Verification items for the finished model (mm, model axes). A direction names the side the tool comes from. Give positions to 0.01 mm unless a question says otherwise; leave off trailing zeros. Loops run counter-clockwise (first coordinate to the right, second up) from the corner with the lowest first, then second, coordinate; pieces in that order, holes last. Notation, with made-up numbers: (-11, 83.25) -> (38, 83.25) arc R37 cw to (38, 120.25) -> close; hole circle Ø11 at (-27.75, 41.5). An arc over 180 degrees is marked (long way). Answer in a Markdown table with one row per item. Add a question column.
Q1. Release check for a two-part mould opening along Y. For faces 1 (the face through (73, 34, 5)), 2 (the face through (-0.86, 56.6, 5.07)), 3 (the face through (86.2, 12.6, 5)) record: pulls with the +Y half, pulls with the -Y half, needs draft (parallel to the pull), parting line crosses it, or undercut.
Q2. Material ranges on probe 1 along X at (y, z) = (13.5, 2); probe 2 along Y at (x, z) = (-11, 6.9); probe 3 along X at (y, z) = (33.5, 5.5), recorded low to high.
Q3. Section check C-C on z = 8. Enter the section's corners in (x, y).
Q4. Section check D-D on z = 1.5. Enter the section's corners in (x, y).
Q5. Gauge pin test, flat ends, axial feed: P1, Ø5, axis at x = -9.5, y = 14.5, coming from the +Z side; P2, Ø4, axis at x = 48, z = 2, coming from the +Y side. Record the tip position at first contact, or that the pin passes through.
Q6. Section check B-B on x = -11. Enter the section's corners in (y, z), and give its area (3 significant figures).
Q7. Section check A-A on y = 39. Enter the section's corners in (x, z).
Q8. Set-up check for faces 4 (the face through (73.9, 0.86, 7.46)), 5 (the face through (-8.69, 9.25, 7.54)), 6 (the face through (-10, 57.5, 5)), 7 (the face through (73.86, 56.6, 5.07)), 8 (the face through (-11.273, 53.265, 5.07)): record each of +Z, -Z, +X, -X, +Y, -Y from which the full face is reachable in a straight line by a thin tool's end or side.
```python
from build123d import *

# Parameters (mm, degrees)
F0_W     = 73
F0_H     = 20
F1_DEPTH = 10
F2_W     = 73
F2_H     = 20
F3_DEPTH = 5
F4_R     = 2.1
F5_DEPTH = 10.001
F6_R     = 5
F6_R_2   = 2.1
F7_DEPTH = 5
F8_R     = 3


with BuildPart() as f1:
    # F0 (on Top) → F1 (new body)
    with BuildSketch(Plane.XY):
        Polygon((-20, 0), (0, 0), (0, 20), (0, 57.5), (-20, 57.5), align=None)
        with Locations((36.5, 10)):
            Rectangle(F0_W, F0_H)
        Polygon((73, 20), (73, 0), (93, 0), (93, 57.5), (73, 57.5), align=None)
    extrude(amount=F1_DEPTH)

    # F2 (on face) → F3 (cut)
    with BuildSketch(Plane.XY.offset(10)):
        with Locations((36.5, 10)):
            Rectangle(F2_W, F2_H)
    extrude(amount=-F3_DEPTH, mode=Mode.SUBTRACT)

    # F4 (on face) → F5 (cut, through all)
    with BuildSketch(Plane.XY.offset(10)):
        with Locations((-11, 13.6832475166)):
            Circle(F4_R)
        with Locations((84, 13.563519451)):
            Circle(F4_R)
        with Locations((-11, 51.1832475166)):
            Circle(F4_R)
        with Locations((84, 51.1832475166)):
            Circle(F4_R)
    extrude(amount=-F5_DEPTH, mode=Mode.SUBTRACT)

    # F6 (on face) → F7 (cut)
    with BuildSketch(Plane.XY.offset(10)):
        with Locations((-11, 13.6832475166)):
            Circle(F6_R)
        with Locations((-11, 13.6832475166)):
            Circle(F6_R_2, mode=Mode.SUBTRACT)
        with Locations((84, 13.6832475166)):
            Circle(F6_R)
    extrude(amount=-F7_DEPTH, mode=Mode.SUBTRACT)

    # F8
    f8_edges = [f1.edges().sort_by_distance(p)[0] for p in [
        (-20, 57.5, 5),
        (0, 57.5, 5),
        (73, 57.5, 5),
        (93, 57.5, 5),
        (-20, 0, 5),
        (93, 0, 5),
        (0, 0, 7.5),
        (73, 0, 7.5),
    ]]
    fillet(f8_edges, radius=F8_R)


solid = f1.part
```
Taken from the geometry:
| question | item | result |
|---|---|---|
| 1 | face 1 | needs draft |
| 1 | face 2 | pulls with the +Y half |
| 1 | face 3 | undercut |
| 2 | probe 1 | x = -20 to -13.09, -8.91 to 81.9, 86.1 to 93 |
| 2 | probe 2 | y = 0 to 8.68, 18.68 to 49.08, 53.28 to 57.5 |
| 2 | probe 3 | x = -20 to 0, 73 to 93 |
| 3 | outline | (-20, 3) arc R3 ccw to (-17, 0) -> (-3, 0) arc R3 ccw to (0, 3) -> (0, 54.5) arc R3 ccw to (-3, 57.5) -> (-17, 57.5) arc R3 ccw to (-20, 54.5) -> close; (73, 3) arc R3 ccw to (76, 0) -> (90, 0) arc R3 ccw to (93, 3) -> (93, 54.5) arc R3 ccw to (90, 57.5) -> (76, 57.5) arc R3 ccw to (73, 54.5) -> close; hole circle Ø10 at (-11, 13.68); hole circle Ø4.2 at (-11, 51.18); hole circle Ø10 at (84, 13.68); hole circle Ø4.2 at (84, 51.18) |
| 4 | outline | (-20, 3) arc R3 ccw to (-17, 0) -> (90, 0) arc R3 ccw to (93, 3) -> (93, 54.5) arc R3 ccw to (90, 57.5) -> (76, 57.5) arc R3 ccw to (73, 54.5) -> (73, 20) -> (0, 20) -> (0, 54.5) arc R3 ccw to (-3, 57.5) -> (-17, 57.5) arc R3 ccw to (-20, 54.5) -> close; hole circle Ø4.2 at (-11, 13.68); hole circle Ø4.2 at (-11, 51.18); hole circle Ø4.2 at (84, 13.56); hole circle Ø4.2 at (84, 51.18) |
| 5 | P1 | stops at z = 5 |
| 5 | P2 | stops at y = 20 |
| 6 | outline | (0, 0) -> (11.58, 0) -> (11.58, 5) -> (8.68, 5) -> (8.68, 10) -> (0, 10) -> close; (15.78, 0) -> (49.08, 0) -> (49.08, 10) -> (18.68, 10) -> (18.68, 5) -> (15.78, 5) -> close; (53.28, 0) -> (57.5, 0) -> (57.5, 10) -> (53.28, 10) -> close |
| 6 | area | 462 mm² |
| 7 | outline | (-20, 0) -> (0, 0) -> (0, 10) -> (-20, 10) -> close; (73, 0) -> (93, 0) -> (93, 10) -> (73, 10) -> close |
| 8 | face 4 | +Z, -Y |
| 8 | face 5 | +Z |
| 8 | face 6 | +Z, -Z, +X, -X, +Y |
| 8 | face 7 | +Z, -Z, +Y |
| 8 | face 8 | +Z, -Z |
